Read the model definition and answer for the solid it produces. Units are mm, in the model's axes. Coordinates: 2 decimals unless noted, no trailing zeros. Write each loop counter-clockwise with the first axis right and the second up, starting at its lowest first coordinate (ties: lowest second). Pieces come first, ordered by that corner, then holes.
1) The part is cut by section C-C (x = -34). Determine the outline of the cut face in (y, z).
2) This flat-tipped pin is pushed along its axis until it touches: pin 1 Ø1 at (x, y) = (-38.5, -0.5) entering from +Z. Where does it stop, or does it pass through?
3) The part is cut by section B-B (z = 2.5). Determine the outline of the cut face in (x, y), then the cut area to 3 significant figures.
4) The part is cut by section A-A (y = 1). Determine the outline of the cut face in (x, z), then the cut area to 3 significant figures.
5) Find the intervals of material crossed by line 1 (Z direction, x = -34.5, y = 3.25), in increasing order.
from build123d import *

# Parameters (mm, degrees)
F0_W        = 50
F0_H        = 8.5
F1_DEPTH    = 5
F2_SIZE2    = 4.6630765815
F2_SIZE     = 10
F3_T1_DEPTH = 67.7710723862


# Not quite as in the source:
# - a fillet or chamfer that OpenCascade refuses, or shapes differently, is made with other operations: its cross-section is extruded or revolved along the edge and cut away or added
# - a feature of the source that left no trace in its solid (it failed there, or was rolled back) is left out


with BuildPart() as f1:
    # F0 (on Top) → F1 (new body)
    with BuildSketch(Plane.XY):
        with Locations((-25, 0)):
            Rectangle(F0_W, F0_H)
        with Locations((25, 0)):
            Rectangle(F0_W, F0_H)
    extrude(amount=F1_DEPTH)

    # F2
    f2_edges = [f1.edges().sort_by_distance(p)[0] for p in [
        (-50, 0, 5),
    ]]
    f2_side = f1.faces().sort_by_distance((0, 0, 5))[0]
    chamfer(f2_edges, length=F2_SIZE, length2=F2_SIZE2, reference=f2_side)

    # F3: fillet of radius 53.5430809348 on 1 edges, made by hand

    # F3_s2 → F3_t1 (cut)
    with BuildSketch(Plane.XZ.offset(-33.8855361931)):
        with BuildLine():
            ThreePointArc((-50, 0.3369234184), (-39.3188667185, 3.8212559042), (-28.1457855228, 5))
            Line((-28.1457855228, 5), (-40, 5))
            Line((-40, 5), (-50, 0.3369234184))
        make_face()
    extrude(amount=F3_T1_DEPTH, mode=Mode.SUBTRACT)


solid = f1.part
Reported:
1. outline: (-4.25, 0) - (4.25, 0) - (4.25, 4.68) - (-4.25, 4.68) - close
2. pin 1: stops at z = 4.09
3. outline: (-44.32, -4.25) - (50, -4.25) - (50, 4.25) - (-44.32, 4.25) - close
3. area: 802 mm2
4. outline: (-50, 0) - (50, 0) - (50, 5) - (-28.15, 5) arc R53.54 ccw to (-50, 0.34) - close
4. area: 467 mm2
5. line 1: z = 0 to 4.62
